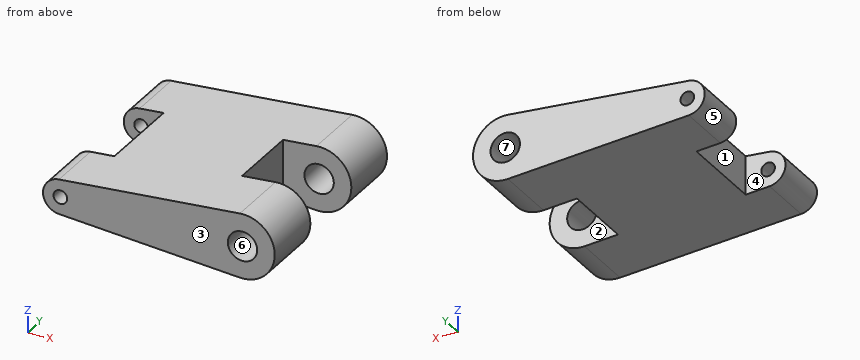
```python
from build123d import *

# Parameters (mm, degrees)
EXTRUDE2_DEPTH          = 11.304095629
CUT_EXTRUDE5_DEPTH      = 26.221647195
CUT_EXTRUDE5_DEPTH_BACK = 26.221647195
SKETCH4_W               = 7.62
SKETCH4_H               = 8.252337146
SKETCH5_R               = 1.64
CUT_EXTRUDE6_DEPTH      = 32.929284696
EXTRUDE4_DEPTH          = 26.221647195
EXTRUDE4_DEPTH_BACK     = 26.221647195
SKETCH6_W               = 4.445
SKETCH6_H               = 9.908191258
SKETCH7_R               = 0.762
EXTRUDE5_DEPTH          = 32.929284696


with BuildPart() as part:
    # Sketch2 → Extrude2 (new, symmetric)
    with BuildSketch(Plane(origin=(0.008589011, 0, 0), x_dir=(1, 0, 0), z_dir=(0, 1, 0))):
        with BuildLine():
            Line((-0.302201676, 3.58467598), (-20.486785806, 1.931402555))
            ThreePointArc((-20.486785806, 1.931402555), (-22.266459506, 0), (-20.486785806, -1.931402555))
            Line((-20.486785806, -1.931402555), (-0.302201676, -3.58467598))
            ThreePointArc((-0.302201676, -3.58467598), (3.588091442, 0), (-0.302201676, 3.58467598))
        make_face()
    extrude(amount=EXTRUDE2_DEPTH, both=True)

    # Sketch4 → Cut-Extrude5 (cut, two sides: drawn at the far end of the back side and taken through both)
    with BuildSketch(Plane.XY.offset(-CUT_EXTRUDE5_DEPTH_BACK)):
        with Locations((-0.213319547, 0)):
            Rectangle(SKETCH4_W, SKETCH4_H)
    extrude(amount=CUT_EXTRUDE5_DEPTH + CUT_EXTRUDE5_DEPTH_BACK, mode=Mode.SUBTRACT)

    # Sketch5 → Cut-Extrude6 (cut, through all)
    with BuildSketch(Plane.XZ.offset(11.304095629)):
        with Locations(Location((0, 0, 0), (0, 0, 270))):
            Circle(SKETCH5_R)
    extrude(amount=-CUT_EXTRUDE6_DEPTH, mode=Mode.SUBTRACT)

    # Sketch6 → Extrude4 (cut, two sides: drawn at the far end of the back side and taken through both)
    with BuildSketch(Plane.XY.offset(-EXTRUDE4_DEPTH_BACK)):
        with Locations((-20.035370495, 0)):
            Rectangle(SKETCH6_W, SKETCH6_H)
    extrude(amount=EXTRUDE4_DEPTH + EXTRUDE4_DEPTH_BACK, mode=Mode.SUBTRACT)

    # Sketch7 → Extrude5 (cut, through all)
    with BuildSketch(Plane.XZ.offset(11.304095629)):
        with Locations(Location((-20.32, 0, 0), (0, 0, 270))):
            Circle(SKETCH7_R)
    extrude(amount=-EXTRUDE5_DEPTH, mode=Mode.SUBTRACT)


solid = part.part
```
Check sheet for the modelled part. Datum: model origin and axes. Units: mm. Face numbers are marked on the shaded views. A direction names the side the tool comes from. Coordinates: 2 decimals unless noted, no trailing zeros. Loops run counter-clockwise (first coordinate to the right, second up) from the corner with the lowest first, then second, coordinate; pieces in that order, holes last. Notation, with made-up numbers: M 63.25,-32 L 122.25,-32 A19 ccw 122.25,5 Z; hole C 15,83 d3. An arc over 180 degrees is marked long. Answer as a JSON object with one key per item and string values.
1. Sectioned sample at A-A on x = 0. Record the cut outline in (y, z), and give its area (3 significant figures).
Outcome:
{"outline": "M -11.3,-3.6 L -4.13,-3.6 L -4.13,-1.64 L -11.3,-1.64 Z; M -11.3,1.64 L -4.13,1.64 L -4.13,3.6 L -11.3,3.6 Z; M 4.13,-3.6 L 11.3,-3.6 L 11.3,-1.64 L 4.13,-1.64 Z; M 4.13,1.64 L 11.3,1.64 L 11.3,3.6 L 4.13,3.6 Z", "area": "56.2 mm²"}
2. Scan lines: L1, parallel to X at y = -4, z = -1.25; L2, parallel to X at y = 6, z = -1.5; L3, parallel to Z at x = -13.25, y = -0.75. Record each from-to range of solid material in increasing order. Write a range as from..to.
Outcome:
{"L1": "-17.81..-4.02", "L2": "-21.55..-0.66, 0.66..3.27", "L3": "-2.52..2.52"}
3. Depth check by flat-ended pin: P1, Ø2, axis at y = -1, z = -1, coming from the +X side; P2, Ø2, axis at x = -7.5, y = 0.5, coming from the +Z side; P3, Ø6, axis at x = -14, y = -1.5, coming from the +Z side; P4, Ø3, axis at x = 0, z = 0, coming from the -Y side. Enter the tip coordinate at first touch or a pass-through.
Outcome:
{"P1": "x = -4.02", "P2": "z = 3.08", "P3": "z = 2.71", "P4": "through"}
4. Release check for a two-part mould opening along X. For the marked faces 4, 5, 6 and 7 record: pulls with the +X half, pulls with the -X half, needs draft (parallel to the pull), parting line crosses it, or undercut.
Outcome:
{"face 4": "needs draft", "face 5": "pulls with the -X half", "face 6": "undercut", "face 7": "undercut"}
5. Sectioned sample at C-C on y = -7. Record the cut outline in (x, z).
Outcome:
{"outline": "M -20.48,-1.93 L -0.29,-3.58 A3.6 ccw long -0.29,3.58 L -20.48,1.93 A1.94 ccw Z; hole C -20.32,0 d1.52; hole C 0,0 d3.28"}
6. Sectioned sample at D-D on z = -2.5. Record the cut outline in (x, y), and give its area (3 significant figures).
Outcome:
{"outline": "M -13.54,-11.3 L 2.59,-11.3 L 2.59,-4.13 L -4.02,-4.13 L -4.02,4.13 L 2.59,4.13 L 2.59,11.3 L -13.54,11.3 Z", "area": "310 mm²"}
7. Sectioned sample at B-B on z = 0. Record the cut outline in (x, y), and give its area (3 significant figures).
Outcome:
{"outline": "M -22.26,-11.3 L -21.08,-11.3 L -21.08,-4.95 L -22.26,-4.95 Z; M -22.26,4.95 L -21.08,4.95 L -21.08,11.3 L -22.26,11.3 Z; M -19.56,-11.3 L -1.64,-11.3 L -1.64,-4.13 L -4.02,-4.13 L -4.02,4.13 L -1.64,4.13 L -1.64,11.3 L -19.56,11.3 L -19.56,4.95 L -17.81,4.95 L -17.81,-4.95 L -19.56,-4.95 Z; M 1.64,-11.3 L 3.6,-11.3 L 3.6,-4.13 L 1.64,-4.13 Z; M 1.64,4.13 L 3.6,4.13 L 3.6,11.3 L 1.64,11.3 Z", "area": "411 mm²"}
8. Access from +Z, -Z, +X, -X, +Y, -Y to the whole of each face (thin tool, end or side, straight path). Record for the marked faces 1, 2 and 3.
Outcome:
{"face 1": "+Z, -Z, -X", "face 2": "+Z, -Z, +X", "face 3": "+Z, -Z, +X, -X, -Y"}
